Design review of the part built by this model. Coordinates are the model's own, in mm. Give positions to 0.01 mm unless a question says otherwise; leave off trailing zeros. Loops run counter-clockwise (first coordinate to the right, second up) from the corner with the lowest first, then second, coordinate; pieces in that order, holes last. Notation, with made-up numbers: (-2.5, 34.25) - (18.5, 34.25) arc R20 ccw to (18.5, 40.25) - close; hole circle Ø2 at (37, 5). An arc over 180 degrees is marked (long way). Write each question's results on one line, items separated by ' | '.
Autodesk Inventor part; units mm, degrees
ref_plane "YZ Plane" through (0, 0, 0) normal (1, 0, 0) x (0, 1, 0)
ref_plane "XZ Plane" through (0, 0, 0) normal (0, 1, 0) x (-1, 0, 0)
ref_plane "XY Plane" through (0, 0, 0) normal (0, 0, 1) x (1, 0, 0)
sketch "Sketch1" plane through (0, 0, 0) normal (1, 0, 0) x (0, 1, 0)
  line L0 (0, 0) -> (0, -101.6)
  arc A0 (0, -101.6) -> (10.2089, -139.7) centre (76.2, -101.6) ccw
  line L1 (10.2089, -139.7) -> (61.0089, -227.6882)
  dimension "bendAngleSketch" = 150
  dimension "CLR" = 76.2
  dimension "ST" = 101.6
sketch "Sketch2" plane through (0, 0, 0) normal (0, 0, 1) x (1, 0, 0)
  circle A0 centre (0, 0) radius 12.7
  circle A1 centre (0, 0) radius 9.652
  dimension "outerDiameter" = 25.4
  dimension "wallThickness" = 3.048
sweep "Sweep1" add profiles "Sketch2" path "Sketch1"
equation "\"bendAngle\" = 30deg"
properties part number "TB11GA1330"
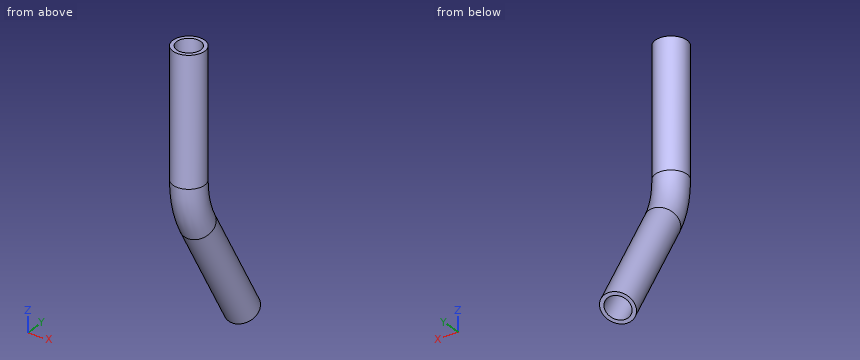
Item 1: Wall thickness on probe 1 along X at (y, z) = (0, -33); probe 2 along Y at (x, z) = (7, -212): over which ranges is each line inside the solid? List them lowest first.
Output values:
probe 1: x = -12.7 to -9.65, 9.65 to 12.7 | probe 2: y = 39.72 to 44.28, 59.62 to 64.19
Item 2: Clearance check with flat-ended pins moving along their axes: P1, Ø5, axis at x = -2.5, z = -198.5, coming from the -Y side; P2, Ø4, axis at x = 6, z = -32, coming from the -Y side; P3, Ø4, axis at x = 2.5, z = -72.5, coming from the -Y side. State where each tip first meets the part, or that it passes through.
Output values:
P1: stops at y = 28.25 | P2: stops at y = -12.05 | P3: stops at y = -12.69
Item 3: We need section A-A on z = -30. Give the boundary of the cut face in (x, y), then the cut area to 3 significant figures.
Output values:
outline: circle Ø25.4 at (0, 0); hole circle Ø19.3 at (0, 0) | area: 214 mm²
